Autodesk Inventor part; units mm, degrees
ref_plane "YZ Plane" through (0, 0, 0) normal (1, 0, 0) x (0, 1, 0)
ref_plane "XZ Plane" through (0, 0, 0) normal (0, 1, 0) x (-1, 0, 0)
ref_plane "XY Plane" through (0, 0, 0) normal (0, 0, 1) x (1, 0, 0)
sketch "Skizze1" plane through (0, 0, 0) normal (0, 0, 1) x (1, 0, 0)
  line L0 (-15, -15) -> (15, -15)
  line L1 (15, -15) -> (15, 15)
  line L2 (15, 15) -> (-15, 15)
  line L3 (-15, 15) -> (-15, -15)
  line L4 (-15, -15) -> (15, 15) construction
  line L5 (15, -15) -> (-15, 15) construction
  point P0 (0, 0)
  dimension "d0" = 30
  dimension "d1" = 30
extrude "Extrusion1" add sketch "Skizze1" along normal blind 1
sketch "Sketch2" plane through (0, 0, 1) normal (0, 0, 1) x (1, 0, 0)
  line L0 (-15, -15) -> (15, -15) construction
  line L1 (15, -15) -> (15, 15) construction
  line L2 (15, 15) -> (-15, 15) construction
  line L3 (-15, 15) -> (-15, -15) construction
  line L4 (-7.535, 7.535) -> (7.535, 7.535) construction
  line L5 (7.535, 7.535) -> (7.535, -7.535) construction
  line L6 (7.535, -7.535) -> (-7.535, -7.535) construction
  line L7 (-7.535, -7.535) -> (-7.535, 7.535) construction
  point P0 (0, 0)
  dimension "d4" = 7.465
hole "Hole1" at (-7.535, 7.535, 1) at (7.535, 7.535, 1) at (7.535, -7.535, 1) at (-7.535, -7.535, 1) direction (0, 0, -1) diameter 2.93 end through all
equation "\"d1\" = d0"
properties part number "00_LED-ARRAY_4x4"
Build history of the part. All positions in model axes, mm. Give positions to 0.01 mm unless a question says otherwise; leave off trailing zeros. Loops run counter-clockwise (first coordinate to the right, second up) from the corner with the lowest first, then second, coordinate; pieces in that order, holes last.
Item 1: Pull direction X, two halves, no side cores. Call faces 1 (the face through (7.47, -6.07, 0.49)), 2 (the face through (0, 0, 1)), 3 (the face through (-15, 0.2, 0.5)): released by +X, released by -X, zero draft, split by the parting line, or undercut.
Answers follow:
face 1: undercut
face 2: zero draft
face 3: released by -X
Item 2: Slice it at A-A, the plane z = 0.85. List the corners of the cut face in (x, y) (3 decimals), and give its area (3 significant figures).
Answers follow:
outline: (-15, -15) - (15, -15) - (15, 15) - (-15, 15) - close; hole circle Ø2.93 at (-7.535, -7.535); hole circle Ø2.93 at (-7.535, 7.535); hole circle Ø2.93 at (7.535, -7.535); hole circle Ø2.93 at (7.535, 7.535)
area: 873 mm2
Item 3: Drill centre lines: line 1 (Y direction, x = -7.5, z = 0.65); line 2 (Y direction, x = 6.75, z = 0.9); line 3 (X direction, y = 7.25, z = 0.5). Where is each one in solid material? Low to high.
Answers follow:
line 1: y = -15 to -9, -6.07 to 6.07, 9 to 15
line 2: y = -15 to -8.77, -6.3 to 6.3, 8.77 to 15
line 3: x = -15 to -8.97, -6.1 to 6.1, 8.97 to 15
